from build123d import *

# Parameters (mm, degrees)
SKETCH_2_R                  = 2.9
CUT_EXTRUDE_1_DEPTH         = 3.5
CUT_EXTRUDE_2_REACH         = 17.174
SKETCH_3_R                  = 1.5
HOLE_WIZARD_3_4_3_4_1_D     = 3.4
HOLE_WIZARD_3_4_3_4_1_DEPTH = 10
HOLE_WIZARD_3_4_3_4_1_TIP   = 1.021463052
CHAMFER_1_SIZE              = 0.2


with BuildPart() as part:
    # 草图1 → 旋转1 (revolve)
    with BuildSketch(Plane.XY, mode=Mode.PRIVATE) as revolve_1_sk:
        Polygon((0, 0), (0, 10), (2, 10), (2, 5), (5.5, 5), (5.5, 0), align=None)
    revolve(revolve_1_sk.sketch.rotate(Axis((0, 0, 0), (1, 0, 0)), 90), axis=Axis((0, 0, 0), (1, 0, 0)))

    # 草图2 → 切除-拉伸1 (cut)
    with BuildSketch(Plane(origin=(5.5, 0, 0), x_dir=(0, 0, -1), z_dir=(1, 0, 0))):
        Circle(SKETCH_2_R)
    extrude(amount=-CUT_EXTRUDE_1_DEPTH, mode=Mode.SUBTRACT)

    # 草图3 → 切除-拉伸2 (cut, up to next)
    with BuildSketch(Plane.ZY, mode=Mode.PRIVATE) as cut_extrude_2_sk1:
        Circle(SKETCH_3_R)
    cut_extrude_2_tool1 = extrude(cut_extrude_2_sk1.sketch, amount=-CUT_EXTRUDE_2_REACH, mode=Mode.PRIVATE) & part.part
    add(cut_extrude_2_tool1.solids().sort_by_distance((0, 0, 0))[0], mode=Mode.SUBTRACT)

    # Ø3.4 (3.4) 直径孔1
    with Locations(Plane(origin=(2, 0, 0), x_dir=(0, 0, -1), z_dir=(1, 0, 0))):
        with Locations((0, 7), (0, -7), (-7, 0), (7, 0)):
            Hole(HOLE_WIZARD_3_4_3_4_1_D / 2, depth=HOLE_WIZARD_3_4_3_4_1_DEPTH)
            with Locations((0, 0, -(HOLE_WIZARD_3_4_3_4_1_DEPTH + HOLE_WIZARD_3_4_3_4_1_TIP / 2))):  # 118° drill point
                Cone(0, HOLE_WIZARD_3_4_3_4_1_D / 2, HOLE_WIZARD_3_4_3_4_1_TIP, mode=Mode.SUBTRACT)

    # 倒角1
    chamfer_1_edges = [part.edges().sort_by_distance(p)[0] for p in [
        (5.5, 0, 2.9),
        (0, 0, -1.5),
        (5.5, 0, -5),
        (2, 0, -10),
        (0, 0, -10),
    ]]
    chamfer(chamfer_1_edges, length=CHAMFER_1_SIZE)


solid = part.part
Input: part model. Units: mm. Frame: model coordinates. A direction names the side the tool comes from. Coordinates: 2 decimals unless noted, no trailing zeros. Order: outer loops, then holes, each group sorted by start corner. A loop starts at its lowest first (then second) coordinate and runs counter-clockwise, first axis right, second up.
1. Cut plane B-B, the plane x = 4.85. Return loops of the section in (y, z).
Checked values:
outline: circle Ø10 at (0, 0); hole circle Ø5.8 at (0, 0)
2. Contact query for flat-ended pins moving along their axis: P1, Ø1.7, axis at y = -1, z = 0, coming from the +X side; P2, Ø3, axis at y = -7, z = 0, coming from the -X side; P3, Ø2, axis at x = 0.5, y = -4, coming from the +Z side. Output: stop coordinate, or through.
Checked values:
P1: stops at x = 2
P2: passes through
P3: stops at z = 9.54
3. Access query for faces 4 (the cylindrical face through (0.99, -1.03, 5.65)), 5 (the cylindrical face through (3.7, 0.1, 2.9)). Directions: +Z, -Z, +X, -X, +Y, -Y. A direction counts if a zero-diameter tool reaches every point of the face in a straight line with its end or side. Return the directions, or none.
Checked values:
face 4: +X, -X
face 5: +X
4. Draft query along Y for faces 1 (the cylindrical face through (4, 0, -5)), 2 (the flat face through (0, 0, -2)), 3 (the cylindrical face through (0.99, -1.03, -8.35)). Return one class per face: +Y half, -Y half, draft (parallel to the pull), parting line (faces both ways), or undercut.
Checked values:
face 1: parting line
face 2: draft
face 3: undercut
5. Ray query, line 1 along X through (y, z) = (7.75, 4.5); line 2 along Y through (x, z) = (0.5, -7); line 3 along Z through (x, y) = (0.85, 1.25). Return the intervals inside material, ascending.
Checked values:
line 1: x = 0 to 2
line 2: y = -7.14 to -1.7, 1.7 to 7.14
line 3: z = -9.92 to -8.15, -5.85 to -0.83, 0.83 to 5.85, 8.15 to 9.92
6. Cut plane A-A, the plane y = 0. Count the separate pieces of the cut face and the enclosed holes in it, plus the area to 3 significant figures.
Checked values:
separate pieces: 4
enclosed holes: 0
area: 34.9 mm2
